Model file for the job. Use its own axes, mm. A direction names the side the tool comes from. Round coordinates to 2 decimals unless told otherwise and drop trailing zeros. Order: outer loops, then holes, each group sorted by start corner. A loop starts at its lowest first (then second) coordinate and runs counter-clockwise, first axis right, second up. Notation, with made-up numbers: M 0.5,-31.75 L 10.5,-31.75 A9 ccw 10.5,-25.75 Z; hole C 11.5,78 d10. An arc over 180 degrees is marked long. Return JSON: item names as keys, results as strings. Group by question number.
Item 1: Slice it at D-D on x = 0. Write the cut outline in (y, z).
Item 2: Pin check, flat tips, straight feed: pin 1 Ø3 at (y, z) = (-1.5, 37) entering from +X; pin 2 Ø2.5 at (x, z) = (15, 35) entering from -Y; pin 3 Ø1.6 at (x, z) = (-0.5, 30.5) entering from +Y; pin 4 Ø5.5 at (y, z) = (4.5, 35.5) entering from -X. Stop position of each tip, or through.
Item 3: Pull direction Z, two halves, no side cores. Call faces 1 (the face through (-16.2, 12.5, 35.9)), 2 (the face through (-0.187, -8.498, 34.451)), 3 (the face through (0, 1, 29)), 4 (the face through (12.5, 5, 35)): pulls with the +Z half, pulls with the -Z half, needs draft (parallel to the pull), parting line crosses it, or undercut.
Item 4: Slice it at B-B on y = 3.5. Write the cut outline in (x, z), then the cut area to 3 significant figures.
Item 5: Slice it at C-C on z = 40.25. Write the cut outline in (x, y).
Item 6: Slice it at A-A on x = 15. Write the cut outline in (y, z).
Item 7: Which spindle directions (+Z, -Z, +X, -X, +Y, -Y) get a long thin tool onto all of the face, cutting with end or side? Do faces 5 (the face through (-17, 10.5, 35)), 6 (the face through (-3.5, 7, 39)), 7 (the face through (3.5, 13, 30)). Say none if no direction does.
Item 8: Probe line 1 along X through (y, z) = (11.8, 35); line 2 along X through (y, z) = (2, 33); line 3 along Z through (x, y) = (-7, 12). List the from-to ranges inside material, lowest first.
from build123d import *

# Parameters (mm, degrees)
SALIENTE_EXTRUIR1_DEPTH    = 38
SALIENTE_EXTRUIR2_DEPTH    = 3
SALIENTE_EXTRUIR3_DEPTH    = 2
CROQUIS4_R                 = 1.5
SALIENTE_EXTRUIR4_DEPTH    = 4
CROQUIS5_W                 = 35
CROQUIS5_H                 = 31
CORTAR_EXTRUIR1_DEPTH      = 24
CORTAR_EXTRUIR1_DEPTH_BACK = 5
SALIENTE_EXTRUIR5_DEPTH    = 2


with BuildPart() as part:
    # Croquis1 → Saliente-Extruir1 (new body)
    with BuildSketch(Plane.XY):
        with BuildLine():
            Line((10.5, 10.5), (12.5, 10.5))
            Line((12.5, 10.5), (12.5, 0))
            ThreePointArc((12.5, 0), (0, -12.5), (-12.5, 0))
            Line((-12.5, 0), (-12.5, 10.5))
            Line((-12.5, 10.5), (-10.5, 10.5))
            Line((-10.5, 10.5), (-8.5, 10.5))
            Line((-8.5, 10.5), (-8.5, 0))
            ThreePointArc((-8.5, 0), (0, -8.5), (8.5, 0))
            Line((8.5, 0), (8.5, 10.5))
            Line((8.5, 10.5), (10.5, 10.5))
        make_face()
    extrude(amount=SALIENTE_EXTRUIR1_DEPTH)

    # Croquis2 → Saliente-Extruir2 (add)
    with BuildSketch(Plane.XY.offset(38)):
        with BuildLine():
            Line((-12.5, 10.5), (-3.5, 10.5))
            Line((-3.5, 10.5), (-3.5, 0))
            ThreePointArc((-3.5, 0), (0, -3.5), (3.5, 0))
            Line((3.5, 0), (3.5, 10.5))
            Line((3.5, 10.5), (12.5, 10.5))
            Line((12.5, 10.5), (12.5, 0))
            ThreePointArc((12.5, 0), (0, -12.5), (-12.5, 0))
            Line((-12.5, 0), (-12.5, 10.5))
        make_face()
    extrude(amount=SALIENTE_EXTRUIR2_DEPTH)

    # Croquis3 → Saliente-Extruir3 (add)
    with BuildSketch(Plane(origin=(0, 0, 0), x_dir=(-1, 0, 0), z_dir=(0, 0, -1))):
        with BuildLine():
            Line((-12.5, 10.5), (12.5, 10.5))
            Line((12.5, 10.5), (12.5, 0))
            ThreePointArc((12.5, 0), (0, -12.5), (-12.5, 0))
            Line((-12.5, 0), (-12.5, 10.5))
        make_face()
    extrude(amount=SALIENTE_EXTRUIR3_DEPTH)

    # Croquis4 → Saliente-Extruir4 (add)
    with BuildSketch(Plane(origin=(0, 10.5, 0), x_dir=(1, 0, 0), z_dir=(0, 1, 0))):
        Polygon((17.5, -41), (3.5, -41), (3.5, -38), (8.5, -38), (8.5, -26.565627665), (17.5, -26.565627665), align=None)
        with Locations((15, -35)):
            Circle(CROQUIS4_R, mode=Mode.SUBTRACT)
        Polygon((-17.5, -41), (-17.5, -26.565627665), (-8.5, -26.565627665), (-8.5, -38), (-3.5, -38), (-3.5, -41), align=None)
        with Locations((-15, -35)):
            Circle(CROQUIS4_R, mode=Mode.SUBTRACT)
    extrude(amount=SALIENTE_EXTRUIR4_DEPTH)

    # Croquis5 → Cortar-Extruir1 (cut, two sides)
    with BuildSketch(Plane.XZ.offset(-10.5)) as cortar_extruir1_sk:
        with Locations((0, 13.5)):
            Rectangle(CROQUIS5_W, CROQUIS5_H)
    extrude(amount=CORTAR_EXTRUIR1_DEPTH, mode=Mode.SUBTRACT)
    extrude(cortar_extruir1_sk.sketch, amount=-CORTAR_EXTRUIR1_DEPTH_BACK, mode=Mode.SUBTRACT)

    # Croquis6 → Saliente-Extruir5 (add)
    with BuildSketch(Plane(origin=(0, 0, 29), x_dir=(-1, 0, 0), z_dir=(0, 0, -1))):
        with BuildLine():
            Line((-8.5, 14.5), (-3.5, 14.5))
            Line((-3.5, 14.5), (-3.5, 12.017542708))
            Line((-3.5, 12.017542708), (3.5, 12.017542708))
            Line((3.5, 12.017542708), (3.5, 14.5))
            Line((3.5, 14.5), (8.5, 14.5))
            Line((8.5, 14.5), (8.5, 0))
            ThreePointArc((8.5, 0), (0, -8.5), (-8.5, 0))
            Line((-8.5, 0), (-8.5, 14.5))
        make_face()
    extrude(amount=-SALIENTE_EXTRUIR5_DEPTH)


solid = part.part
Output values:
{
 "1": {"outline": "M -12.5,29 L 12.02,29 L 12.02,31 L -8.5,31 L -8.5,38 L -3.5,38 L -3.5,41 L -12.5,41 Z"},
 "2": {"pin 1": "x = 12.5", "pin 2": "through", "pin 3": "y = 12.02", "pin 4": "x = -12.5"},
 "3": {"face 1": "undercut", "face 2": "undercut", "face 3": "pulls with the -Z half", "face 4": "needs draft"},
 "4": {"outline": "M -12.5,29 L 12.5,29 L 12.5,41 L 3.5,41 L 3.5,38 L 8.5,38 L 8.5,31 L -8.5,31 L -8.5,38 L -3.5,38 L -3.5,41 L -12.5,41 Z", "area": "160 mm²"},
 "5": {"outline": "M -17.5,10.5 L -12.5,10.5 L -12.5,0 A12.5 ccw 12.5,0 L 12.5,10.5 L 17.5,10.5 L 17.5,14.5 L 3.5,14.5 L 3.5,0 A3.5 cw -3.5,0 L -3.5,14.5 L -17.5,14.5 Z"},
 "6": {"outline": "M 10.5,29 L 14.5,29 L 14.5,33.5 L 10.5,33.5 Z; M 10.5,36.5 L 14.5,36.5 L 14.5,41 L 10.5,41 Z"},
 "7": {"face 5": "+Z, -Z, -X, -Y", "face 6": "+Z, +Y", "face 7": "+Z, -Z, +Y"},
 "8": {"line 1": "-17.5 to -16.5, -13.5 to -8.5, 8.5 to 13.5, 16.5 to 17.5", "line 2": "-12.5 to -8.5, 8.5 to 12.5", "line 3": "29 to 31, 38 to 41"}
}
